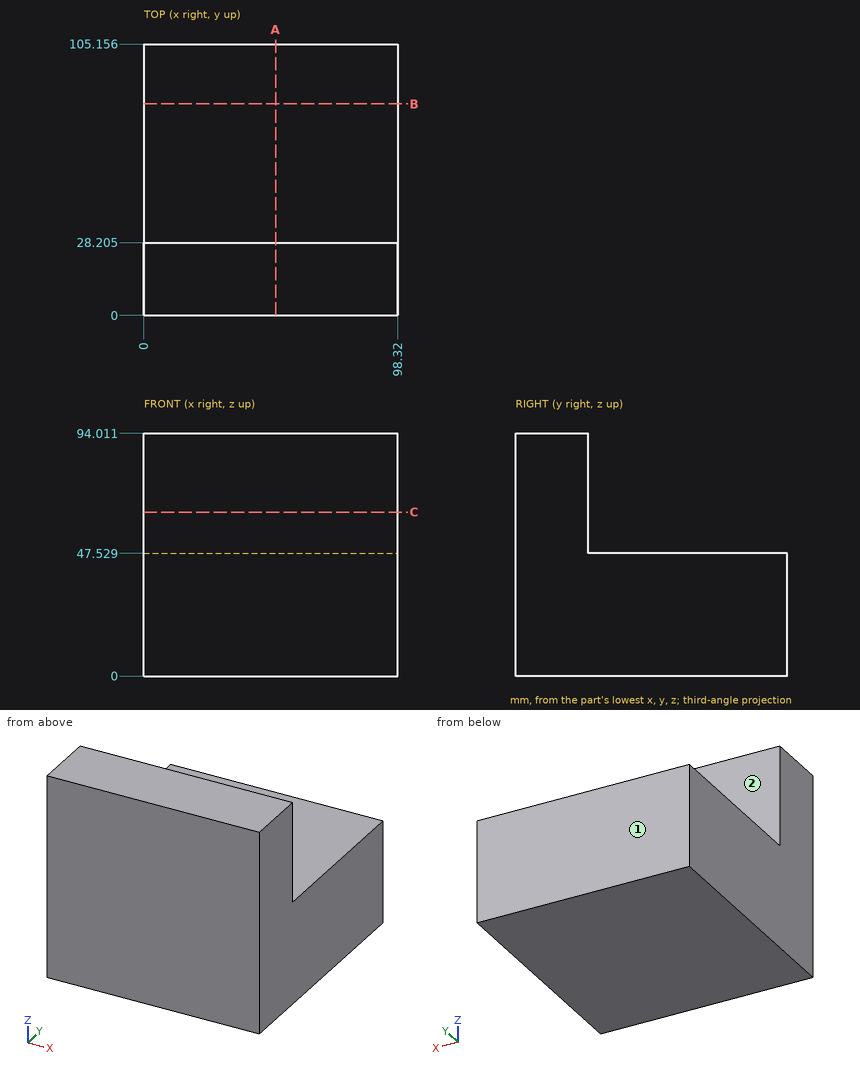
The drawing under review shows one solid part. Ordinate dimensions are in mm from its lowest x, y, z. A direction names the side the tool comes from. Give positions to 0.01 mm unless a question says otherwise; leave off trailing zeros. Order: outer loops, then holes, each group sorted by start corner. A loop starts at its lowest first (then second) coordinate and runs counter-clockwise, first axis right, second up. Notation, with made-up numbers: (-37.5, 7.25) - (13.5, 7.25) arc R9 cw to (13.5, 16.25) - close; hole circle Ø7 at (88, 36). An arc over 180 degrees is marked (long way). Answer as a JSON object with one key per item and string values. Group by question number.
Item 1: Take a section at B-B on y = 82. Give the boundary of the cut face in (x, z).
Item 2: Take a section at C-C on z = 63.5. Give the boundary of the cut face in (x, y) (1 decimal).
Item 3: Wall thickness on line 1 along Z through (x, y) = (27, 60.5); line 2 along Y through (x, z) = (69, 78) (1 decimal): over which ranges is each line inside the solid? List them lowest first.
Item 4: Machinability: for the marked faces 1 and 2, which of the approach directions +Z, -Z, +X, -X, +Y, -Y give a long, thin tool a straight path to every point of the face, cutting with its end or side? Answer none if there is none.
Item 5: Take a section at A-A on x = 51. Give the boundary of the cut face in (y, z) (1 decimal).
Item 6: Clearance check with flat-ended pins moving along their axes: pin 1 Ø5 at (x, z) = (17, 61) entering from +Y (1 decimal); pin 2 Ø1 at (x, y) = (45.5, 54) entering from +Z. State where each tip first meets the part, or that it passes through.
Reported:
{
 "1": {"outline": "(0, 0) - (98.32, 0) - (98.32, 47.53) - (0, 47.53) - close"},
 "2": {"outline": "(0, 0) - (98.3, 0) - (98.3, 28.2) - (0, 28.2) - close"},
 "3": {"line 1": "0 to 47.53", "line 2": "0 to 28.2"},
 "4": {"face 1": "+Z, -Z, +X, -X, +Y", "face 2": "+Z, +X, -X, +Y"},
 "5": {"outline": "(0, 0) - (105.2, 0) - (105.2, 47.5) - (28.2, 47.5) - (28.2, 94) - (0, 94) - close"},
 "6": {"pin 1": "y = 28.2", "pin 2": "z = 47.53"}
}
